from build123d import *

# Parameters (mm, degrees)
BLOCK_OUTLINE_W                            = 6
BLOCK_OUTLINE_H                            = 51.4
REACTION_BLOCK_THICKNESS_DEPTH             = 8.2
LANE_1_INNER_CABLE_CLEARANCE_PROFILE_R     = 1.1
LANE_1_INNER_CABLE_CLEARANCE_DEPTH         = 6.2
LANE_1_COMPRESSION_HOUSING_SOCKET_PROFIL_R = 2.05
LANE_1_COMPRESSION_HOUSING_SOCKET_DEPTH    = 4.1
LANE_2_INNER_CABLE_CLEARANCE_PROFILE_R     = 1.1
LANE_2_INNER_CABLE_CLEARANCE_DEPTH         = 6.2
LANE_2_COMPRESSION_HOUSING_SOCKET_PROFIL_R = 2.05
LANE_2_COMPRESSION_HOUSING_SOCKET_DEPTH    = 4.1
LANE_3_INNER_CABLE_CLEARANCE_PROFILE_R     = 1.1
LANE_3_INNER_CABLE_CLEARANCE_DEPTH         = 6.2
LANE_3_COMPRESSION_HOUSING_SOCKET_PROFIL_R = 2.05
LANE_3_COMPRESSION_HOUSING_SOCKET_DEPTH    = 4.1
M2_FIXING_CLEARANCE_1_PROFILE_R            = 1.1
M2_FIXING_CLEARANCE_1_DEPTH                = 8.4
M2_FIXING_CLEARANCE_2_PROFILE_R            = 1.1
M2_FIXING_CLEARANCE_2_DEPTH                = 8.4


with BuildPart() as part:
    # Block outline → Reaction block thickness (new body)
    with BuildSketch(Plane.XY.offset(11)):
        with Locations((-63.291651246, -29)):
            Rectangle(BLOCK_OUTLINE_W, BLOCK_OUTLINE_H)
    extrude(amount=REACTION_BLOCK_THICKNESS_DEPTH)

    # Lane 1 inner cable clearance profile → Lane 1 inner cable clearance (cut)
    with BuildSketch(Plane(origin=(-66.391651246, 0, 0), x_dir=(0, 0, -1), z_dir=(1, 0, 0))):
        with Locations(Location((-15, -12, 0), (0, 0, 180))):
            Circle(LANE_1_INNER_CABLE_CLEARANCE_PROFILE_R)
    extrude(amount=LANE_1_INNER_CABLE_CLEARANCE_DEPTH, mode=Mode.SUBTRACT)

    # Lane 1 compression housing socket profil → Lane 1 compression housing socket (cut)
    with BuildSketch(Plane(origin=(-66.391651246, 0, 0), x_dir=(0, 0, -1), z_dir=(1, 0, 0))):
        with Locations((-15, -12)):
            Circle(LANE_1_COMPRESSION_HOUSING_SOCKET_PROFIL_R)
    extrude(amount=LANE_1_COMPRESSION_HOUSING_SOCKET_DEPTH, mode=Mode.SUBTRACT)

    # Lane 2 inner cable clearance profile → Lane 2 inner cable clearance (cut)
    with BuildSketch(Plane(origin=(-66.391651246, 0, 0), x_dir=(0, 0, -1), z_dir=(1, 0, 0))):
        with Locations(Location((-15, -29, 0), (0, 0, 180))):
            Circle(LANE_2_INNER_CABLE_CLEARANCE_PROFILE_R)
    extrude(amount=LANE_2_INNER_CABLE_CLEARANCE_DEPTH, mode=Mode.SUBTRACT)

    # Lane 2 compression housing socket profil → Lane 2 compression housing socket (cut)
    with BuildSketch(Plane(origin=(-66.391651246, 0, 0), x_dir=(0, 0, -1), z_dir=(1, 0, 0))):
        with Locations((-15, -29)):
            Circle(LANE_2_COMPRESSION_HOUSING_SOCKET_PROFIL_R)
    extrude(amount=LANE_2_COMPRESSION_HOUSING_SOCKET_DEPTH, mode=Mode.SUBTRACT)

    # Lane 3 inner cable clearance profile → Lane 3 inner cable clearance (cut)
    with BuildSketch(Plane(origin=(-66.391651246, 0, 0), x_dir=(0, 0, -1), z_dir=(1, 0, 0))):
        with Locations(Location((-15, -46, 0), (0, 0, 180))):
            Circle(LANE_3_INNER_CABLE_CLEARANCE_PROFILE_R)
    extrude(amount=LANE_3_INNER_CABLE_CLEARANCE_DEPTH, mode=Mode.SUBTRACT)

    # Lane 3 compression housing socket profil → Lane 3 compression housing socket (cut)
    with BuildSketch(Plane(origin=(-66.391651246, 0, 0), x_dir=(0, 0, -1), z_dir=(1, 0, 0))):
        with Locations((-15, -46)):
            Circle(LANE_3_COMPRESSION_HOUSING_SOCKET_PROFIL_R)
    extrude(amount=LANE_3_COMPRESSION_HOUSING_SOCKET_DEPTH, mode=Mode.SUBTRACT)

    # M2 fixing clearance 1 profile → M2 fixing clearance 1 (cut)
    with BuildSketch(Plane.XY.offset(10.9)):
        with Locations((-63.291651246, -5.5)):
            Circle(M2_FIXING_CLEARANCE_1_PROFILE_R)
    extrude(amount=M2_FIXING_CLEARANCE_1_DEPTH, mode=Mode.SUBTRACT)

    # M2 fixing clearance 2 profile → M2 fixing clearance 2 (cut)
    with BuildSketch(Plane.XY.offset(10.9)):
        with Locations((-63.291651246, -52.5)):
            Circle(M2_FIXING_CLEARANCE_2_PROFILE_R)
    extrude(amount=M2_FIXING_CLEARANCE_2_DEPTH, mode=Mode.SUBTRACT)


solid = part.part
Work out the finished part from the listing and answer in its coordinate system (mm). A direction names the side the tool comes from. Coordinates: 2 decimals unless noted, no trailing zeros. Write each loop counter-clockwise with the first axis right and the second up, starting at its lowest first coordinate (ties: lowest second). Pieces come first, ordered by that corner, then holes.
1. The part is cut by section A-A, the plane y = -12. Write down the section's boundary in (x, z), and give its area (3 significant figures).
Results list:
outline: (-66.29, 11) - (-60.29, 11) - (-60.29, 13.9) - (-62.29, 13.9) - (-62.29, 12.95) - (-66.29, 12.95) - close; (-66.29, 17.05) - (-62.29, 17.05) - (-62.29, 16.1) - (-60.29, 16.1) - (-60.29, 19.2) - (-66.29, 19.2) - close
area: 28.4 mm2
2. The part is cut by section D-D, the plane y = -52.5. Write down the section's boundary in (x, z).
Results list:
outline: (-66.29, 11) - (-64.39, 11) - (-64.39, 19.2) - (-66.29, 19.2) - close; (-62.19, 11) - (-60.29, 11) - (-60.29, 19.2) - (-62.19, 19.2) - close
3. For a pull along Y with two mould halves and no side action, classify faces 1 (the cylindrical face through (-61.306, -27.926, 14.762)), 2 (the cylindrical face through (-64.39, -5.45, 15.04)), 3 (the flat face through (-63, -29, 19.2)), 4 (the flat face through (-63, -54.7, 15)) as +Y half, -Y half, draft (parallel to the pull), parting line (faces both ways), or undercut.
Results list:
face 1: undercut
face 2: undercut
face 3: draft
face 4: -Y half
4. Consider line 1 along Y through (x, z) = (-60.8, 15); line 2 along Y through (x, z) = (-65, 15); line 3 along Y through (x, z) = (-62.95, 15.25). Determine where each line is inside the solid, lowest interval first.
Results list:
line 1: y = -54.7 to -47.1, -44.9 to -30.1, -27.9 to -13.1, -10.9 to -3.3
line 2: y = -54.7 to -48.05, -43.95 to -31.05, -26.95 to -14.05, -9.95 to -3.3
line 3: y = -54.7 to -53.55, -51.45 to -48.03, -43.97 to -31.03, -26.97 to -14.03, -9.97 to -6.55, -4.45 to -3.3
5. The part is cut by section C-C, the plane z = 15. State how many separate pieces and enclosed holes the cut face has, and give its area (3 significant figures).
Results list:
separate pieces: 4
enclosed holes: 2
area: 238 mm2
6. The part is cut by section B-B, the plane x = -63.65. Write down the section's boundary in (y, z).
Results list:
outline: (-54.7, 11) - (-53.54, 11) - (-53.54, 19.2) - (-54.7, 19.2) - close; (-51.46, 11) - (-6.54, 11) - (-6.54, 19.2) - (-51.46, 19.2) - close; (-4.46, 11) - (-3.3, 11) - (-3.3, 19.2) - (-4.46, 19.2) - close; hole circle Ø4.1 at (-46, 15); hole circle Ø4.1 at (-29, 15); hole circle Ø4.1 at (-12, 15)
7. A flat-ended cylindrical pin translates along its axis: pin 1 (2 mm diameter, centred on y = -46, z = 14.5, fed in from -X). Find the tip coordinate at first contact, or state that the pin passes through.
Results list:
pin 1: stops at x = -62.29
8. For faces 5 (the cylindrical face through (-64.32, -13.247, 16.627)), 6 (the flat face through (-60.292, -29, 17)), determine the directions among +Z, -Z, +X, -X, +Y, -Y from which every point of the face is accessible in a straight line to the end or side of a thin tool.
Results list:
face 5: -X
face 6: +Z, -Z, +X, +Y, -Y
